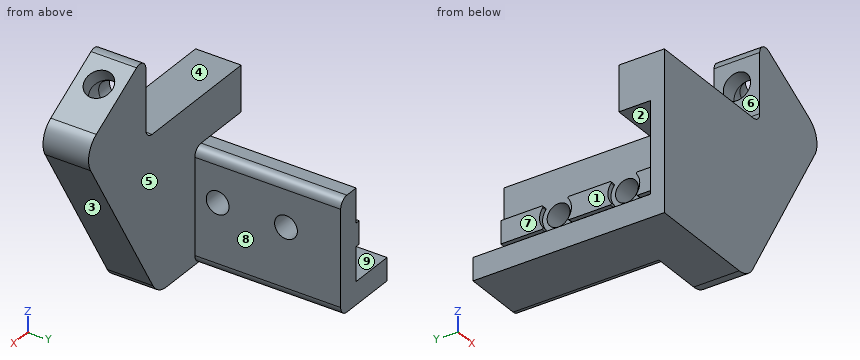
```python
from build123d import *

# Parameters (mm, degrees)
SKETCH1_W                = 20
SKETCH1_H                = 20.000000000000014
BOSS_EXTRUDE1_DEPTH      = 10
SKETCH2_R                = 3.000000000000015
CUT_EXTRUDE1_DEPTH       = 120.06125706799004
BOSS_EXTRUDE2_DEPTH      = 32
BOSS_EXTRUDE2_DEPTH_BACK = 10
SKETCH7_R                = 2.4999999999999956
CUT_EXTRUDE3_DEPTH       = 20
SKETCH8_W                = 10
SKETCH8_H                = 20.000000000000014
BOSS_EXTRUDE4_DEPTH      = 3
BOSS_EXTRUDE5_DEPTH      = 1
FILLET1_R                = 0.25
FILLET3_R                = 2
FILLET4_R                = 5


with BuildPart() as part:
    # Sketch1 → Boss-Extrude1 (new body)
    with BuildSketch(Plane(origin=(0, 0, 0), x_dir=(1, 0, 0), z_dir=(0, 1, 0))):
        Polygon((-51.25019936166113, 65.23205080756885), (-46.92007234273894, 62.732050807568854), (-30.867513459481355, 53.46410161513777), (-30.867513459481355, 72), (30.867513459481284, 72), (30.867513459481284, 53.46410161513781), (46.92007234273889, 62.73205080756891), (51.25019936166109, 65.23205080756892), (27.13546265191245, 106.99999999999991), (-27.135462651912732, 106.99999999999991), align=None)
        with Locations((0, 91.99999999999991)):
            Rectangle(SKETCH1_W, SKETCH1_H, mode=Mode.SUBTRACT)
    extrude(amount=BOSS_EXTRUDE1_DEPTH)

    # Cut-Sweep1: sweep along a path in Sketch3
    with BuildLine(Plane(origin=(0, 5, 0), x_dir=(1, 0, 0), z_dir=(0, 1, 0))) as cut_sweep1_path:
        Line((-30.867513459481355, 62.499999999999986), (-34.35234101678278, 62.499999999999986))
        ThreePointArc((-34.35234101678278, 62.499999999999986), (-35.85234101678278, 62.0980762113533), (-36.9504172281361, 60.999999999999986))
        Line((-36.9504172281361, 60.999999999999986), (-38.69283100678681, 57.98205080756888))
    # Sketch2 → Cut-Sweep1 (sweep, cut)
    with BuildSketch(Plane(origin=(-30.867513459481355, 0, 0), x_dir=(0, 0, -1), z_dir=(1, 0, 0))):
        with Locations((62.49999999999999, 5)):
            Circle(SKETCH2_R)
    cut_sweep1 = sweep(path=cut_sweep1_path.line, mode=Mode.SUBTRACT)

    # Mirror3: Cut-Sweep1 across plane
    add(cut_sweep1.mirror(Plane(origin=(0, 0, 0), x_dir=(0, 0, 1), z_dir=(1, 0, 0))), mode=Mode.SUBTRACT)

    # Sketch4 → Cut-Extrude1 (cut, through all)
    with BuildSketch(Plane(origin=(0, 0, 0), x_dir=(0, 0, -1), z_dir=(1, 0, 0))):
        Polygon((65.23205080756894, 0), (106.99999999999991, 0), (106.99999999999991, 10), (65.23205080756894, 10), (53.46410161513781, 10), (53.46410161513781, 0), align=None)
    extrude(amount=-CUT_EXTRUDE1_DEPTH, mode=Mode.SUBTRACT)

    # Sketch5 → Boss-Extrude2 (add, two sides: drawn at the far end of the back side and taken through both)
    with BuildSketch(Plane(origin=(0, 10, 0), x_dir=(1, 0, 0), z_dir=(0, 1, 0)).offset(-BOSS_EXTRUDE2_DEPTH_BACK)):
        Polygon((10, 81.99999999999991), (10, 101.99999999999993), (0, 101.99999999999993), (0, 106.99999999999991), (14.999999999999993, 106.99999999999991), (14.999999999999996, 81.99999999999991), align=None)
    extrude(amount=BOSS_EXTRUDE2_DEPTH + BOSS_EXTRUDE2_DEPTH_BACK)

    # Sketch7 → Cut-Extrude3 (cut)
    with BuildSketch(Plane(origin=(10, 0, 0), x_dir=(0, 0, -1), z_dir=(1, 0, 0))):
        with Locations((91.99999999999991, 15)):
            Circle(SKETCH7_R)
        with Locations((91.99999999999991, 30)):
            Circle(SKETCH7_R)
    extrude(amount=CUT_EXTRUDE3_DEPTH, mode=Mode.SUBTRACT)

    # Sketch8 → Boss-Extrude4 (add)
    with BuildSketch(Plane.XZ):
        with Locations((5, -91.99999999999991)):
            Rectangle(SKETCH8_W, SKETCH8_H)
    extrude(amount=-BOSS_EXTRUDE4_DEPTH)

    # Sketch9 → Boss-Extrude5 (add)
    with BuildSketch(Plane.ZY.offset(-10)):
        with BuildLine():
            Line((-94.49999999999991, 3), (-94.49999999999991, 12.550510257216839))
            ThreePointArc((-94.49999999999991, 12.550510257216839), (-91.99999999999991, 11.500000000000012), (-89.49999999999991, 12.550510257216839))
            Line((-89.49999999999991, 12.550510257216839), (-89.49999999999991, 3.000000000000001))
            Line((-89.49999999999991, 3.000000000000001), (-94.49999999999991, 3))
        make_face()
        with BuildLine():
            Line((-89.49999999999993, 42), (-94.49999999999991, 42))
            Line((-94.49999999999991, 42), (-94.49999999999991, 32.44948974278316))
            ThreePointArc((-94.49999999999991, 32.44948974278316), (-91.99999999999991, 33.499999999999986), (-89.49999999999991, 32.44948974278316))
            Line((-89.49999999999991, 32.44948974278316), (-89.49999999999993, 42))
        make_face()
        with BuildLine():
            Line((-94.49999999999991, 17.44948974278316), (-94.49999999999991, 27.55051025721684))
            ThreePointArc((-94.49999999999991, 27.55051025721684), (-91.9999999999999, 26.50000000000001), (-89.4999999999999, 27.550510257216853))
            Line((-89.4999999999999, 27.550510257216853), (-89.49999999999991, 17.44948974278316))
            ThreePointArc((-89.49999999999991, 17.44948974278316), (-91.99999999999991, 18.49999999999999), (-94.49999999999991, 17.44948974278316))
        make_face()
    extrude(amount=BOSS_EXTRUDE5_DEPTH)

    # Fillet1
    fillet1_edges = [part.edges().sort_by_distance(p)[0] for p in [
        (9.5, 12.550510257216839, -89.49999999999991),
        (9.5, 12.550510257216839, -94.49999999999991),
        (9.5, 32.44948974278316, -94.49999999999991),
        (9.5, 32.44948974278316, -89.49999999999991),
        (9.5, 27.550510257216853, -89.4999999999999),
        (9.5, 27.55051025721684, -94.49999999999991),
        (9.5, 17.44948974278316, -94.49999999999991),
        (9.5, 17.44948974278316, -89.49999999999991),
    ]]
    fillet(fillet1_edges, radius=FILLET1_R)

    # Fillet3
    fillet3_edges = [part.edges().sort_by_distance(p)[0] for p in [
        (14.999999999999996, 26, -81.99999999999991),
        (14.999999999999993, 26, -106.99999999999991),
        (30.867513459481284, 5, -53.46410161513781),
        (30.867513459481284, 5, -72),
    ]]
    fillet(fillet3_edges, radius=FILLET3_R)

    # Fillet4
    fillet4_edges = [part.edges().sort_by_distance(p)[0] for p in [
        (27.135462651912448, 5, -106.99999999999991),
        (51.2501993616611, 5, -65.23205080756894),
    ]]
    fillet(fillet4_edges, radius=FILLET4_R)


solid = part.part
```
The listing builds one solid part. Answer for the finished solid, in the listing's coordinates (mm). Face numbers are marked on the shaded views. A direction names the side the tool comes from. Give positions to 0.01 mm unless a question says otherwise; leave off trailing zeros. Order: outer loops, then holes, each group sorted by start corner. A loop starts at its lowest first (then second) coordinate and runs counter-clockwise, first axis right, second up. Notation, with made-up numbers: M -21,44 L 30,44 A35 cw 30,83 Z; hole C 43,31.25 d9. An arc over 180 degrees is marked long. Put each result on its own line as item: value. Start each with the question number.
Item 1: The part is cut by section C-C, the plane y = 25. Determine the outline of the cut face in (x, z).
Item 2: The part is cut by section D-D, the plane x = 22. Determine the outline of the cut face in (y, z).
Item 3: For a pull along Z with two mould halves and no side action, classify the marked faces 1, 2, 3 and 4 as +Z half, -Z half, draft (parallel to the pull), parting line (faces both ways), or undercut.
Item 4: Which of the six approach directions +Z, -Z, +X, -X, +Y, -Y give full straight-line access (tool end or side, diameter ignored) to the marked faces 5, 6, 7, 8 and 9?
Item 5: The part is cut by section A-A, the plane y = 30. Determine the outline of the cut face in (x, z), and give its area (3 significant figures).
Item 6: Find the intervals of material crossed by line 1 along Y through (x, z) = (11, -92); line 2 along Y through (x, z) = (33.5, -62.5); line 3 along Z through (x, y) = (13.05, 15), in increasing order.
Item 7: Flat-ended cylindrical pins translate along their axes: P1, Ø4, axis at y = 23.5, z = -87.5, coming from the +X side; P2, Ø5, axis at x = 6, z = -92, coming from the +Y side; P3, Ø8, axis at x = 11.5, y = 6.5, coming from the +Z side; P4, Ø8, axis at x = 42, z = -83, coming from the -Y side. Find the tip coordinate at first contact, or state that the pin passes through.
Item 8: The part is cut by section B-B, the plane z = -91. Determine the outline of the cut face in (x, y), and give its area (3 significant figures).
Answer key:
1. outline: M 0,-107 L 13,-107 A2 ccw 15,-105 L 15,-84 A2 ccw 13,-82 L 10,-82 L 10,-89.5 L 9,-89.5 L 9,-94.5 L 10,-94.5 L 10,-102 L 0,-102 Z
2. outline: M 0,-107 L 10,-107 L 10,-72 L 0,-72 Z
3. face 1: draft
3. face 2: undercut
3. face 3: -Z half
3. face 4: +Z half
4. face 5: +Z, +X, +Y
4. face 6: +Z, -X, +Y, -Y
4. face 7: +Z, -X, +Y
4. face 8: +Z, -Z, +X, +Y
4. face 9: -X, +Y
5. outline: M 0,-107 L 13,-107 A2 ccw 15,-105 L 15,-94.5 L 10,-94.5 L 10,-102 L 0,-102 Z; M 10,-89.5 L 15,-89.5 L 15,-84 A2 ccw 13,-82 L 10,-82 Z
5. area: 148 mm²
6. line 1: y = 0 to 12.5, 17.5 to 27.5, 32.5 to 42
6. line 2: y = 0 to 2, 8 to 10
6. line 3: z = -107 to -94.5, -89.5 to -82
7. P1: stops at x = 15
7. P2: stops at y = 3
7. P3: stops at z = -72
7. P4: stops at y = 0
8. outline: M 0,0 L 36.37,0 L 36.37,10 L 15,10 L 15,12.71 L 10,12.71 L 10,11.65 L 9,11.65 L 9,3 L 0,3 Z; M 9,18.35 L 10,18.35 L 10,17.29 L 15,17.29 L 15,27.71 L 10,27.71 L 10,26.65 L 9,26.65 Z; M 9,33.35 L 10,33.35 L 10,32.29 L 15,32.29 L 15,42 L 9,42 Z
8. area: 433 mm²
